```python
from build123d import *

# Parameters (mm, degrees)
SKETCH1_W                      = 4.5
SKETCH1_H                      = 8.85
F_5_2_5_2_DIAMETER_HOLE1_D     = 5.2
F_5_2_5_2_DIAMETER_HOLE1_DEPTH = 8.35
BOSS_EXTRUDE1_DEPTH            = 5.98
BOSS_EXTRUDE2_DEPTH            = 5.98
SKETCH6_R                      = 1.25
BOSS_EXTRUDE3_DEPTH            = 16.852002855
SKETCH7_R                      = 1.25
BOSS_EXTRUDE4_DEPTH            = 0.877097074
BOSS_EXTRUDE4_TAPER            = -54.943518707
SKETCH8_R                      = 2.5
BOSS_EXTRUDE5_DEPTH            = 0.25
CHAMFER1_SIZE                  = 1
FILLET1_R                      = 0.36


with BuildPart() as part:
    # Sketch1 → Revolve1 (revolve)
    with BuildSketch(Plane.XY):
        with Locations((2.25, 4.575)):
            Rectangle(SKETCH1_W, SKETCH1_H)
    revolve(axis=Axis((0, 9, 0), (0, -1, 0)))

    # Ø5.2 (5.2) Diameter Hole1
    with Locations(Plane(origin=(0, 0.15, 0), x_dir=(-1, 0, 0), z_dir=(0, -1, 0))):
        with Locations((0, 0)):
            Hole(F_5_2_5_2_DIAMETER_HOLE1_D / 2, depth=F_5_2_5_2_DIAMETER_HOLE1_DEPTH)

    # Sketch4 → Boss-Extrude1 (add)
    with BuildSketch(Plane.XZ.offset(-8.5)):
        with BuildLine():
            Line((-2, -1.661324773), (2, -1.661324773))
            ThreePointArc((2, -1.661324773), (0, -2.6), (-2, -1.661324773))
        make_face()
    extrude(amount=BOSS_EXTRUDE1_DEPTH)

    # Sketch5 → Boss-Extrude2 (add)
    with BuildSketch(Plane.XZ.offset(-8.5)):
        with BuildLine():
            Line((2, 1.661324773), (-2, 1.661324773))
            ThreePointArc((-2, 1.661324773), (0, 2.6), (2, 1.661324773))
        make_face()
    extrude(amount=BOSS_EXTRUDE2_DEPTH)

    # Sketch6 → Boss-Extrude3 (add)
    with BuildSketch(Plane(origin=(0, 9, 0), x_dir=(-1, 0, 0), z_dir=(0, 1, 0))):
        Circle(SKETCH6_R)
    extrude(amount=BOSS_EXTRUDE3_DEPTH)

    # Sketch7 → Boss-Extrude4 (add)
    with BuildSketch(Plane(origin=(0, 25.852002855, 0), x_dir=(-1, 0, 0), z_dir=(0, 1, 0))):
        Circle(SKETCH7_R)
    extrude(amount=BOSS_EXTRUDE4_DEPTH, taper=BOSS_EXTRUDE4_TAPER)

    # Sketch8 → Boss-Extrude5 (add)
    with BuildSketch(Plane(origin=(0, 26.729099929, 0), x_dir=(-1, 0, 0), z_dir=(0, 1, 0))):
        Circle(SKETCH8_R)
    extrude(amount=BOSS_EXTRUDE5_DEPTH)

    # Chamfer1
    chamfer1_edges = [part.edges().sort_by_distance(p)[0] for p in [
        (-4.5, 9, 0),
    ]]
    chamfer(chamfer1_edges, length=CHAMFER1_SIZE)

    # Fillet1
    fillet1_edges = [part.edges().sort_by_distance(p)[0] for p in [
        (1.25, 9, 0),
    ]]
    fillet(fillet1_edges, radius=FILLET1_R)


solid = part.part
```
Here's how the part is built. I have some questions about the finished solid (model axes, mm). A direction names the side the tool comes from. Give positions to 0.01 mm unless a question says otherwise; leave off trailing zeros. Loops run counter-clockwise (first coordinate to the right, second up) from the corner with the lowest first, then second, coordinate; pieces in that order, holes last. Notation, with made-up numbers: M 69,51.25 L 126,51.25 A29 cw 126,80.25 Z; hole C 80.25,-34 d10. An arc over 180 degrees is marked long. Put each result on its own line as item: value. Start each with the question number.
(1) I want a section at A-A on x = 0. Please give me the cut outline in (y, z).
(2) For faces 1 (the flat face through (0, 6, -1.661)), 2 (the cylindrical face through (-0.59, 4.13, 4.46)), 3 (the flat face through (-1, 9, -2)), which set-ups out of +Z, -Z, +X, -X, +Y, -Y let a thin tool reach every point of the face, with its end or its side?
(3) I need wall thicknesses on line 1 along Z through (x, y) = (0, 6); line 2 along Y through (x, z) = (-2.5, -1.5); line 3 along Z through (x, y) = (0, 22.75). Which ranges of each line are inside material? Lowest first, please. Write a range as [from, to].
(4) If we mould it in two halves opening along Z, with no side actions, what happens to faces 4 (the flat face through (0, 26.979, 0)), 5 (the flat face through (0, 2.52, 2)), 6 (the cylindrical face through (0.27, 17.49, -1.22))? For each: +Z half, -Z half, draft (parallel to the pull), parting line (faces both ways), or undercut.
(5) Will these pins go through, and if not, where does the flat tip stop? pin 1 Ø2.5 at (x, z) = (-1, 0) entering from -Y; pin 2 Ø0.5 at (x, z) = (0.5, -2) entering from -Y; pin 3 Ø1.5 at (x, y) = (-0.5, 16.5) entering from +Z.
(6) I want a section at B-B on y = 15.25. Please give me the cut outline in (x, z).
Answer block:
1. outline: M 0.15,-4.5 L 8,-4.5 L 9,-3.5 L 9,-1.61 A0.36 cw 9.36,-1.25 L 25.85,-1.25 L 26.73,-2.5 L 26.98,-2.5 L 26.98,2.5 L 26.73,2.5 L 25.85,1.25 L 9.36,1.25 A0.36 cw 9,1.61 L 9,3.5 L 8,4.5 L 0.15,4.5 L 0.15,2.6 L 2.52,2.6 L 2.52,1.66 L 8.5,1.66 L 8.5,-1.66 L 2.52,-1.66 L 2.52,-2.6 L 0.15,-2.6 Z
2. face 1: -Y
2. face 2: +Y, -Y
2. face 3: none
3. line 1: [-4.5, -1.66], [1.66, 4.5]
3. line 2: [0.15, 9]
3. line 3: [-1.25, 1.25]
4. face 4: draft
4. face 5: undercut
4. face 6: parting line
5. pin 1: y = 8.5
5. pin 2: y = 2.52
5. pin 3: z = 1.25
6. outline: C 0,0 d2.5
